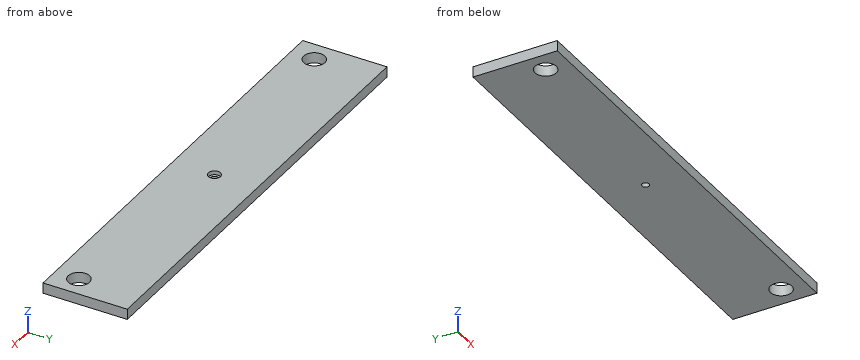
```python
from build123d import *

# Parameters (mm, degrees)
SKETCH1_W           = 812.8
SKETCH1_H           = 152.4
BOSS_EXTRUDE1_DEPTH = 19.05
SKETCH2_R           = 19.2405
CUT_EXTRUDE1_DEPTH  = 19.05
SKETCH3_R           = 10.9982
CUT_EXTRUDE2_DEPTH  = 6.985
SKETCH4_R           = 6.35
CUT_EXTRUDE3_DEPTH  = 828.052092812


with BuildPart() as part:
    # Sketch1 → Boss-Extrude1 (new body)
    with BuildSketch(Plane.XY):
        with Locations((406.4, 76.2)):
            Rectangle(SKETCH1_W, SKETCH1_H)
    extrude(amount=BOSS_EXTRUDE1_DEPTH)

    # Sketch2 → Cut-Extrude1 (cut)
    with BuildSketch(Plane.XY.offset(19.05)):
        with Locations((38.1, 42.926)):
            Circle(SKETCH2_R)
        with Locations((774.7, 42.926)):
            Circle(SKETCH2_R)
    extrude(amount=-CUT_EXTRUDE1_DEPTH, mode=Mode.SUBTRACT)

    # Sketch3 → Cut-Extrude2 (cut)
    with BuildSketch(Plane.XY.offset(19.05)):
        with Locations((406.4, 75.2094)):
            Circle(SKETCH3_R)
    extrude(amount=-CUT_EXTRUDE2_DEPTH, mode=Mode.SUBTRACT)

    # Sketch4 → Cut-Extrude3 (cut, through all)
    with BuildSketch(Plane.XY.offset(12.065)):
        with Locations((406.4, 75.2094)):
            Circle(SKETCH4_R)
    extrude(amount=-CUT_EXTRUDE3_DEPTH, mode=Mode.SUBTRACT)


solid = part.part
```
CAD build for the part. Positions are in the model's coordinates, mm. Give positions to 0.01 mm unless a question says otherwise; leave off trailing zeros. Loops run counter-clockwise (first coordinate to the right, second up) from the corner with the lowest first, then second, coordinate; pieces in that order, holes last. Notation, with made-up numbers: (10.5, 51.25) -> (59.5, 51.25) arc R29 ccw to (59.5, 88.25) -> close; hole circle Ø2 at (46, 54.25). An arc over 180 degrees is marked (long way). Use a Markdown table: item, result.
1. Wall check: L1, parallel to X at y = 76.5, z = 14.25; L2, parallel to Y at x = 38.1, z = 7.75; L3, parallel to X at y = 33.5, z = 4.5. Give the ranges that are in metal, low to high. Write a range as [from, to].
Check result:
| item | result |
|---|---|
| L1 | x = [0, 395.48], [417.32, 812.8] |
| L2 | y = [0, 23.69], [62.17, 152.4] |
| L3 | x = [0, 21.33], [54.87, 757.93], [791.47, 812.8] |
2. Slice it at A-A (x = 774.7). List the corners of the cut face in (y, z), plus the area to 3 significant figures.
Check result:
| item | result |
|---|---|
| outline | (0, 0) -> (23.69, 0) -> (23.69, 19.05) -> (0, 19.05) -> close; (62.17, 0) -> (152.4, 0) -> (152.4, 19.05) -> (62.17, 19.05) -> close |
| area | 2,170 mm^2 |
3. Slice it at C-C (z = 4.5). List the corners of the cut face in (x, y), plus the area to 3 significant figures.
Check result:
| item | result |
|---|---|
| outline | (0, 0) -> (812.8, 0) -> (812.8, 152.4) -> (0, 152.4) -> close; hole circle Ø38.48 at (38.1, 42.93); hole circle Ø12.7 at (406.4, 75.21); hole circle Ø38.48 at (774.7, 42.93) |
| area | 121,000 mm^2 |
4. Slice it at B-B (y = 55.5). List the corners of the cut face in (x, z), plus the area to 3 significant figures.
Check result:
| item | result |
|---|---|
| outline | (0, 0) -> (23.54, 0) -> (23.54, 19.05) -> (0, 19.05) -> close; (52.66, 0) -> (760.14, 0) -> (760.14, 19.05) -> (52.66, 19.05) -> close; (789.26, 0) -> (812.8, 0) -> (812.8, 19.05) -> (789.26, 19.05) -> close |
| area | 14,400 mm^2 |
5. Flat gauge pin, fed straight in: pin 1 (7.5 mm diameter, centred on x = 406.4, y = 75.21, fed in from -Z). Where does the tip first touch, or does it go through?
Check result:
| item | result |
|---|---|
| pin 1 | passes through |
